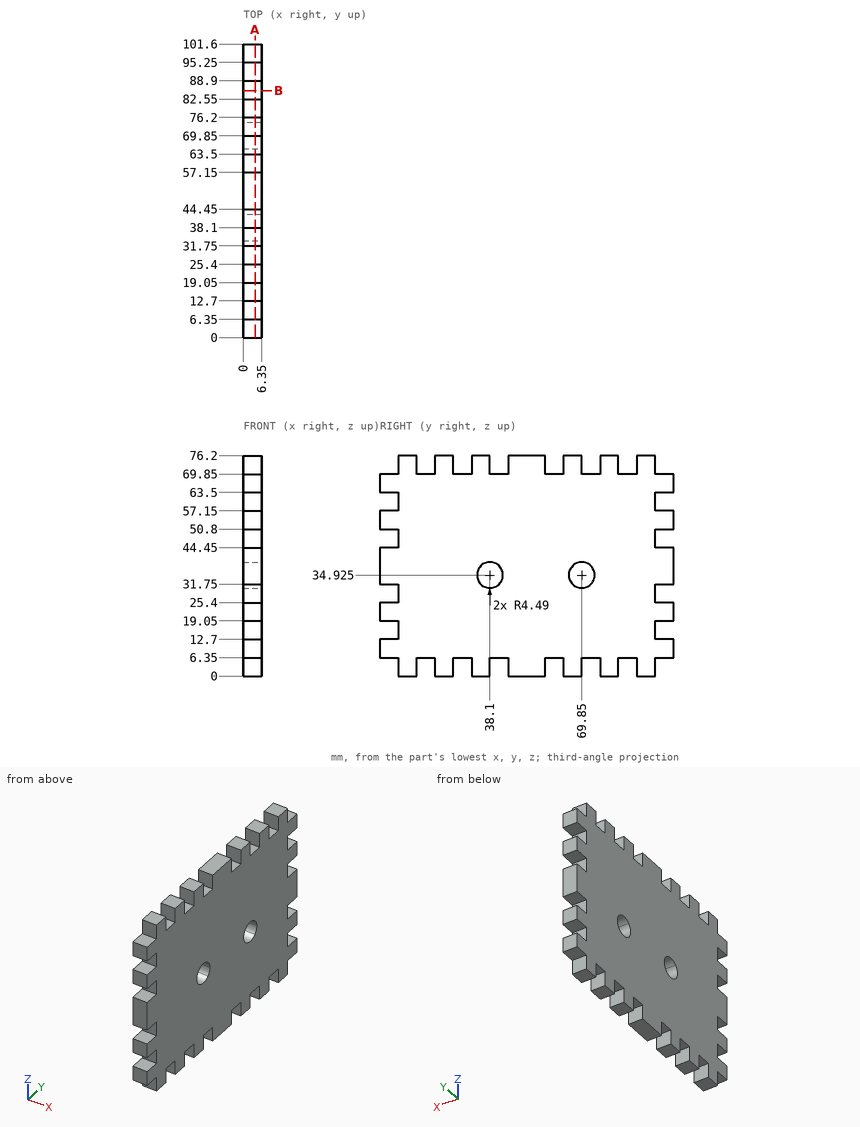
Source: three-view drawing plus pictorial views. Frame: mm from the lowest corner of the part. Round coordinates to 2 decimals unless told otherwise and drop trailing zeros. Loops run counter-clockwise (first coordinate to the right, second up) from the corner with the lowest first, then second, coordinate; pieces in that order, holes last. Notation, with made-up numbers: (12.5, -15.5) - (44.5, -15.5) arc R8 ccw to (44.5, -0.5) - close; hole circle Ø3 at (5.25, 67.5). An arc over 180 degrees is marked (long way). Write item = value, one per line. Start each with the question number.
Item 1: Section query B-B on y = 85.5. Output: boundary loops of the cut face in (x, z), plus the area to 3 significant figures.
Item 2: First-contact query: pin 1 Ø3 at (x, z) = (3.5, 3.5) entering from +Y; pin 2 Ø3 at (x, z) = (3, 72.5) entering from -Y; pin 3 Ø3 at (x, y) = (3, 4.5) entering from -Z. Flat tips, straight axial feed; report the tip coordinate or a pass-through.
Item 3: Section query A-A on x = 4. Count the separate pieces of the cut face and the enclosed holes in it, plus the area to 3 significant figures.
Item 4: Material intervals for line 1 (Z direction, x = 4.25, y = 38); line 2 (Y direction, x = 5.5, z = 50.5); line 3 (Z direction, x = 1.5, y = 29), sorted ascending.
Results list:
q1.outline = (0, 6.35) - (6.35, 6.35) - (6.35, 69.85) - (0, 69.85) - close
q1.area = 403 mm²
q2.pin_1 = 95.25
q2.pin_2 = 6.35
q2.pin_3 = 6.35
q3.separate_pieces = 1
q3.enclosed_holes = 2
q3.area = 6,650 mm²
q4.line_1 = 0 to 30.44, 39.41 to 76.2
q4.line_2 = 6.35 to 95.25
q4.line_3 = 6.35 to 69.85
